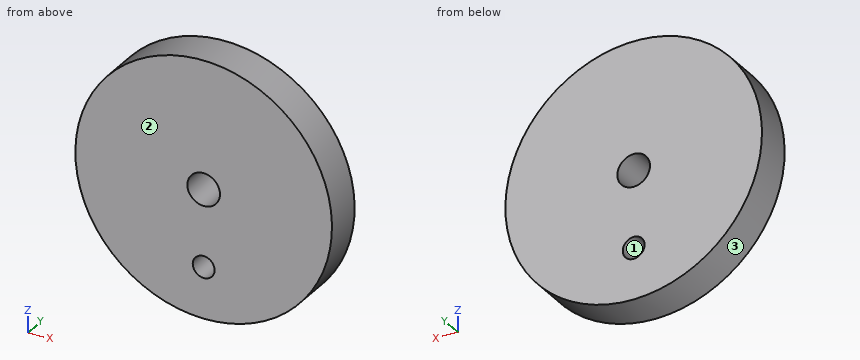
```python
from build123d import *

# Parameters (mm, degrees)
SKETCH1_R              = 15.875
BOSS_EXTRUDE1_DEPTH    = 4.7625
F_10_32_TAPPED_HOLE1_D = 4.0386
F_6_32_TAPPED_HOLE1_D  = 2.7051


with BuildPart() as part:
    # Sketch1 → Boss-Extrude1 (new body)
    with BuildSketch(Plane(origin=(0, 0, 0), x_dir=(1, 0, 0), z_dir=(0, 1, 0))):
        with Locations(Location((0, 0, 0), (0, 0, 90))):
            Circle(SKETCH1_R)
    extrude(amount=BOSS_EXTRUDE1_DEPTH)

    # #10-32 Tapped Hole1 (through all)
    with Locations(Plane(origin=(0, 4.7625, 0), x_dir=(1, 0, 0), z_dir=(0, 1, 0))):
        with Locations((0, 0)):
            Hole(F_10_32_TAPPED_HOLE1_D / 2)

    # #6-32 Tapped Hole1 (through all)
    with Locations(Plane(origin=(0, 4.7625, 0), x_dir=(1, 0, 0), z_dir=(0, 1, 0))):
        with Locations((0, 9.525)):
            Hole(F_6_32_TAPPED_HOLE1_D / 2)


solid = part.part
```
Read the model definition and answer for the solid it produces. Units are mm, in the model's axes. Face numbers are marked on the shaded views. Coordinates: 2 decimals unless noted, no trailing zeros. Loops run counter-clockwise (first coordinate to the right, second up) from the corner with the lowest first, then second, coordinate; pieces in that order, holes last. Notation, with made-up numbers: (6.5, 80) - (51.5, 80) arc R26 cw to (51.5, 111) - close; hole circle Ø5 at (15, 34.5). An arc over 180 degrees is marked (long way). Answer in a Markdown table with one row per item.
1. Given pin 1 (2 mm diameter, centred on x = 8, y = 3, fed in from -Z), flat-ended and moving along its own axis, determine where the tip first touches the part or whether it passes through.
Conclusion:
| item | result |
|---|---|
| pin 1 | stops at z = -14.25 |
2. Straight lines are drawn through the part: line 1 (Z direction, x = 0.5, y = 2.1); line 2 (Z direction, x = 1, y = 1.5); line 3 (X direction, y = 0.85, z = -0.5). For each, find the intervals that lie inside material, in ascending order.
Conclusion:
| item | result |
|---|---|
| line 1 | z = -15.87 to -10.78, -8.27 to -1.96, 1.96 to 15.87 |
| line 2 | z = -15.84 to -10.44, -8.61 to -1.75, 1.75 to 15.84 |
| line 3 | x = -15.87 to -1.96, 1.96 to 15.87 |
3. Find section D-D, the plane x = 4. Write down the section's boundary in (y, z).
Conclusion:
| item | result |
|---|---|
| outline | (0, -15.36) - (4.76, -15.36) - (4.76, 15.36) - (0, 15.36) - close |
4. Find section B-B, the plane y = 1.55. Write down the section's boundary in (x, z) (3 decimals), then the cut area to 3 significant figures.
Conclusion:
| item | result |
|---|---|
| outline | circle Ø31.75 at (0, 0); hole circle Ø4.039 at (0, 0); hole circle Ø2.705 at (0, -9.525) |
| area | 773 mm² |
5. Determine the mould class of the marked faces 1, 2 and 3 for opening direction Z: +Z half, -Z half, draft (parallel to the pull), parting line (faces both ways), or undercut.
Conclusion:
| item | result |
|---|---|
| face 1 | undercut |
| face 2 | draft |
| face 3 | parting line |
6. Find section C-C, the plane z = -13. Write down the section's boundary in (x, y).
Conclusion:
| item | result |
|---|---|
| outline | (-9.11, 0) - (9.11, 0) - (9.11, 4.76) - (-9.11, 4.76) - close |
7. Find section A-A, the plane x = 0. Write down the section's boundary in (y, z) (1 decimal), then the cut area to 3 significant figures.
Conclusion:
| item | result |
|---|---|
| outline | (0, -15.9) - (4.8, -15.9) - (4.8, -10.9) - (0, -10.9) - close; (0, -8.2) - (4.8, -8.2) - (4.8, -2) - (0, -2) - close; (0, 2) - (4.8, 2) - (4.8, 15.9) - (0, 15.9) - close |
| area | 119 mm² |
